```python
from build123d import *

# Parameters (mm, degrees)
ESQUISSE1_W                  = 75
ESQUISSE1_H                  = 70
ESQUISSE1_R                  = 1.5
ESQUISSE1_W_2                = 15
ESQUISSE1_H_2                = 3
BOSS_EXTRU_1_DEPTH           = 3
ENL_V_MAT_EXTRU_2_DEPTH      = 10
ENL_V_MAT_EXTRU_2_DEPTH_BACK = 10


with BuildPart() as part:
    # Esquisse1 → Boss.-Extru.1 (new body)
    with BuildSketch(Plane.XY):
        with Locations((-12.683673469, -2.836734694)):
            Rectangle(ESQUISSE1_W, ESQUISSE1_H)
        with Locations((-38.683673469, 25.663265306)):
            Circle(ESQUISSE1_R, mode=Mode.SUBTRACT)
        with Locations((-38.683673469, 12.663265306)):
            Circle(ESQUISSE1_R, mode=Mode.SUBTRACT)
        with Locations((13.316326531, 12.663265306)):
            Circle(ESQUISSE1_R, mode=Mode.SUBTRACT)
        with Locations((-38.683673469, -32.836734694)):
            Circle(ESQUISSE1_R, mode=Mode.SUBTRACT)
        with Locations((13.316326531, -32.836734694)):
            Circle(ESQUISSE1_R, mode=Mode.SUBTRACT)
        with Locations((7.316326531, 25.663265306)):
            Rectangle(ESQUISSE1_W_2, ESQUISSE1_H_2, mode=Mode.SUBTRACT)
    extrude(amount=BOSS_EXTRU_1_DEPTH)

    # Esquisse2 → Enlèv. mat.-Extru.2 (cut, two sides: drawn at the far end of the back side and taken through both)
    with BuildSketch(Plane.XY.offset(-ENL_V_MAT_EXTRU_2_DEPTH_BACK)):
        Polygon((24.816326531, -1.336734694), (18.816326531, -1.336734694), (18.816326531, -0.311734694), (16.766326531, -0.311734694), (16.766326531, -1.336734694), (10.816326531, -1.336734694), (10.816326531, -4.336734694), (16.766326531, -4.336734694), (16.766326531, -5.361734694), (18.816326531, -5.361734694), (18.816326531, -4.336734694), (24.816326531, -4.336734694), align=None)
        Polygon((-50.183673469, -1.336734694), (-50.183673469, -4.336734694), (-44.183673469, -4.336734694), (-44.183673469, -5.361734694), (-42.133673469, -5.361734694), (-42.133673469, -4.336734694), (-36.183673469, -4.336734694), (-36.183673469, -1.336734694), (-42.133673469, -1.336734694), (-42.133673469, -0.311734694), (-44.183673469, -0.311734694), (-44.183673469, -1.336734694), align=None)
    extrude(amount=ENL_V_MAT_EXTRU_2_DEPTH + ENL_V_MAT_EXTRU_2_DEPTH_BACK, mode=Mode.SUBTRACT)


solid = part.part
```
Check sheet for the modelled part. Datum: model origin and axes. Units: mm. A direction names the side the tool comes from. Give positions to 0.01 mm unless a question says otherwise; leave off trailing zeros. Write each loop counter-clockwise with the first axis right and the second up, starting at its lowest first coordinate (ties: lowest second). Pieces come first, ordered by that corner, then holes. Notation, with made-up numbers: (-11, 40.5) - (-5, 40.5) arc R27 cw to (-5, 61.5) - close; hole circle Ø8 at (-23, 10.25). An arc over 180 degrees is marked (long way). Answer as a JSON object with one key per item and string values. Group by question number.
1) Depth check by flat-ended pin: P1, Ø1.5, axis at y = -2.5, z = 1.5, coming from the -X side; P2, Ø2.5, axis at x = -38.68, y = 25.66, coming from the -Z side. Enter the tip coordinate at first touch or a pass-through.
2) Sectioned sample at A-A (x = 13). Record the cut outline in (y, z), then the cut area to 3 significant figures.
3) Release check for a two-part mould opening along X. For faces 1 (the face through (14.816, 26, 1)), 2 (the face through (-47, -1.337, 1)), 3 (the face through (-36.184, -3, 1)) record: pulls with the +X half, pulls with the -X half, needs draft (parallel to the pull), parting line crosses it, or undercut.
4) Thickness scan on probe 1 along Y at (x, z) = (-40.5, 0.45); probe 2 along Y at (x, z) = (-43, 1.9); probe 3 along X at (y, z) = (25, 2.3). Record the ranges inside material, lowest first. Write a range as from..to.
5) Access from +Z, -Z, +X, -X, +Y, -Y to the whole of each face (thin tool, end or side, straight path). Record for faces 4 (the face through (-0.184, 26, 1)), 5 (the face through (24.816, 15, 1)), 6 (the face through (14, -1.337, 1)), 7 (the face through (-39, -4.337, 1)).
6) Sectioned sample at B-B (z = 0.7). Give the number of separate pieces and of enclosed holes in the cut face, then the cut area to 3 significant figures.
Geometry results:
{
 "1": {"P1": "stops at x = -36.18", "P2": "passes through"},
 "2": {"outline": "(-37.84, 0) - (-34.3, 0) - (-34.3, 3) - (-37.84, 3) - close; (-31.37, 0) - (-4.34, 0) - (-4.34, 3) - (-31.37, 3) - close; (-1.34, 0) - (11.2, 0) - (11.2, 3) - (-1.34, 3) - close; (14.13, 0) - (24.16, 0) - (24.16, 3) - (14.13, 3) - close; (27.16, 0) - (32.16, 0) - (32.16, 3) - (27.16, 3) - close", "area": "174 mm^2"},
 "3": {"face 1": "undercut", "face 2": "needs draft", "face 3": "pulls with the -X half"},
 "4": {"probe 1": "y = -37.84..-4.34, -1.34..32.16", "probe 2": "y = -37.84..-5.36, -0.31..32.16", "probe 3": "x = -50.18..-40.03, -37.34..-0.18, 14.82..24.82"},
 "5": {"face 4": "+Z, -Z", "face 5": "+Z, -Z, +X, +Y, -Y", "face 6": "+Z, -Z, +X", "face 7": "+Z, -Z, -X"},
 "6": {"separate pieces": "1", "enclosed holes": "6", "area": "5,080 mm^2"}
}
